Read the model definition and answer for the solid it produces. Units are mm, in the model's axes. Face numbers are marked on the shaded views. A direction names the side the tool comes from. Give positions to 0.01 mm unless a question says otherwise; leave off trailing zeros. Loops run counter-clockwise (first coordinate to the right, second up) from the corner with the lowest first, then second, coordinate; pieces in that order, holes last. Notation, with made-up numbers: (29.25, 2) -> (52.25, 2) arc R22 cw to (52.25, 30) -> close; hole circle Ø6 at (61.25, 22). An arc over 180 degrees is marked (long way). Return JSON: item names as keys, results as strings. Group by question number.
from build123d import *

# Parameters (mm, degrees)
F0_W     = 11
F0_H     = 7
F1_DEPTH = 4.5
F2_W     = 4
F2_H     = 4
F3_DEPTH = 15
F5_DEPTH = 4
F7_DEPTH = 25
F8_SIZE  = 1
F9_SIZE  = 0.25


with BuildPart() as f1:
    # F0 (on Top) → F1 (new body)
    with BuildSketch(Plane.XY):
        Rectangle(F0_W, F0_H)
    extrude(amount=-F1_DEPTH)

    # F2 (on face) → F3 (join)
    with BuildSketch(Plane.XY):
        Rectangle(F2_W, F2_H)
    extrude(amount=F3_DEPTH)

    # F4 (on face) → F5 (join)
    with BuildSketch(Plane.YZ.offset(2)):
        Polygon((-1.137265, 12.942829), (-1.5, 15), (-4.263235, 2), (-3.463235, 2), align=None)
        Polygon((3.463235, 2), (4.263235, 2), (1.5, 15), (1.137265, 12.942829), align=None)
    extrude(amount=-F5_DEPTH)

    # F6 (on face) → F7 (cut)
    with BuildSketch(Plane.YZ.offset(2)):
        Polygon((-1.33767, 12), (-2, 8.883981), (-2, 2), (-1.33767, 2), align=None)
        Polygon((-1.33767, 2), (-2, 2), (-2, 0), align=None)
        Polygon((2, 2), (2, 8.883981), (1.33767, 12), (1.33767, 2), align=None)
        Polygon((2, 0), (2, 2), (1.33767, 2), align=None)
    extrude(amount=-F7_DEPTH, mode=Mode.SUBTRACT)

    # F8
    f8_edges = [f1.edges().sort_by_distance(p)[0] for p in [
        (-2, 0, 15),
        (0, 2, 15),
        (2, 0, 15),
        (0, -2, 15),
    ]]
    chamfer(f8_edges, length=F8_SIZE)

    # F9
    f9_edges = [f1.edges().sort_by_distance(p)[0] for p in [
        (2, -2, 13.323842),
        (2, -3.131618, 7.323842),
        (-2, -3.131618, 7.323842),
        (-2, -2, 13.323842),
        (-2, 3.131618, 7.323842),
        (-2, 2, 13.323842),
        (2, 2, 13.323842),
        (2, 3.131618, 7.323842),
    ]]
    chamfer(f9_edges, length=F9_SIZE)


solid = f1.part
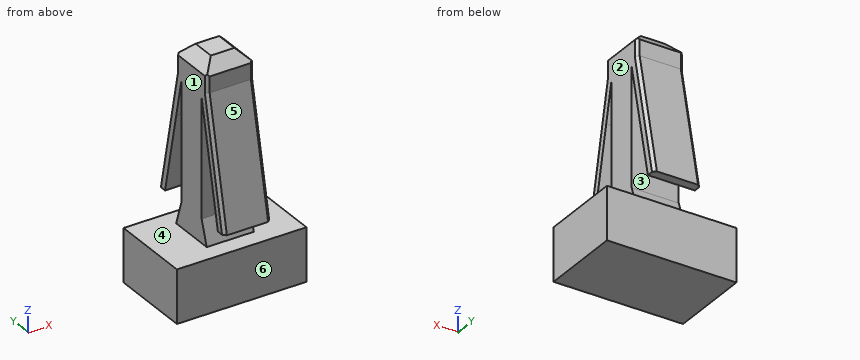
1. Section D-D on x = 2.5 is taken. Determine the outline of the cut face in (y, z).
2. Straight lines are drawn through the part: line 1 (Y direction, x = 0, z = 10.75); line 2 (Y direction, x = 1.5, z = 11.25); line 3 (Y direction, x = -4, z = -2.5). For each, find the intervals that lie inside material, in ascending order. Write a range as from..to.
3. Section C-C on y = -0.75 is taken. Determine the outline of the cut face in (x, z).
4. Section B-B on y = 3 is taken. Determine the outline of the cut face in (x, z), then the cut area to 3 significant figures.
5. Flat-ended cylindrical pins translate along their axes: pin 1 Ø2.5 at (y, z) = (-1.5, 5) entering from +X; pin 2 Ø1 at (x, z) = (3.5, -1.5) entering from -Y; pin 3 Ø0.9 at (x, y) = (-1, -4) entering from -Z. Find the tip coordinate at first contact, or state that the pin passes through.
6. Determine the mould class of the marked faces 4, 5 and 6 for opening direction Z: pulls with the +Z half, pulls with the -Z half, needs draft (parallel to the pull), parting line crosses it, or undercut.
7. Section A-A on z = 10.75 is taken. Determine the outline of the cut face in (x, y), then the cut area to 3 significant figures.
8. Which of the six approach directions +Z, -Z, +X, -X, +Y, -Y give full straight-line access (tool end or side, diameter ignored) to the marked faces 1, 2 and 3?
Completed:
{
 "1": {"outline": "(-3.5, -4.5) -> (3.5, -4.5) -> (3.5, 0) -> (-3.5, 0) -> close"},
 "2": {"line 1": "y = -2.4..-1.6, -1.34..1.34, 1.6..2.4", "line 2": "y = -2.3..-1.5, -1.34..1.34, 1.5..2.3", "line 3": "y = -3.5..3.5"},
 "3": {"outline": "(-5.5, -4.5) -> (5.5, -4.5) -> (5.5, 0) -> (2, 0) -> (2, 14) -> (1, 15) -> (-1, 15) -> (-2, 14) -> (-2, 0) -> (-5.5, 0) -> close"},
 "4": {"outline": "(-5.5, -4.5) -> (5.5, -4.5) -> (5.5, 0) -> (-5.5, 0) -> close; (-2, 4.18) -> (2, 4.18) -> (2, 6.74) -> (1.75, 7.94) -> (-1.75, 7.94) -> (-2, 6.74) -> close", "area": "64.3 mm²"},
 "5": {"pin 1": "stops at x = 2", "pin 2": "stops at y = -3.5", "pin 3": "stops at z = 2"},
 "6": {"face 4": "undercut", "face 5": "pulls with the +Z half", "face 6": "needs draft"},
 "7": {"outline": "(-2, -2.15) -> (-1.75, -2.4) -> (1.75, -2.4) -> (2, -2.15) -> (2, -1.6) -> (-2, -1.6) -> close; (-2, -1.34) -> (2, -1.34) -> (2, 1.34) -> (-2, 1.34) -> close; (-2, 1.6) -> (2, 1.6) -> (2, 2.15) -> (1.75, 2.4) -> (-1.75, 2.4) -> (-2, 2.15) -> close", "area": "17.0 mm²"},
 "8": {"face 1": "+Z, -X, +Y, -Y", "face 2": "+Z, +X, +Y, -Y", "face 3": "+X, -X"}
}
